```python
from build123d import *

# Parameters (mm, degrees)
F0_R     = 3.175
F1_DEPTH = 25.4


with BuildPart() as f1:
    # F0 (on Front) → F1 (new body)
    with BuildSketch(Plane.XZ):
        with BuildLine():
            Line((0.6773435479, -9.500885786), (0, -9.525))
            ThreePointArc((0, -9.525), (0.3388863295, -9.5189695375), (0.6773435479, -9.500885786))
        make_face()
        with BuildLine():
            Line((-15.7942028036, 61.9003804205), (-9.525, 0))
            ThreePointArc((-9.525, 0), (-6.7351920908, 6.7351920908), (0, 9.525))
            Line((0, 9.525), (0, 47.625))
            ThreePointArc((0, 47.625), (-10.644756084, 51.722700101), (-15.7942028036, 61.9003804205))
        make_face()
        with BuildLine():
            ThreePointArc((9.525, 0), (6.9705567315, -6.4912990883), (0.6773435479, -9.500885786))
            Line((0.6773435479, -9.500885786), (44.7324052746, -7.9324746146))
            ThreePointArc((44.7324052746, -7.9324746146), (38.9380895153, -5.7116327839), (36.5125, 0))
            Line((36.5125, 0), (9.525, 0))
        make_face()
        with BuildLine():
            Line((0, 100.0252), (0, 79.375))
            ThreePointArc((0, 79.375), (10.5003255158, 75.40625), (15.7504882737, 65.484375))
            Line((15.7504882737, 65.484375), (9.4502929642, 115.490625))
            ThreePointArc((9.4502929642, 115.490625), (9.5063048942, 114.896483242), (9.525, 114.3))
            ThreePointArc((9.525, 114.3), (6.7351920908, 107.5648079092), (0, 104.775))
            Line((0, 104.775), (0, 100.0252))
        make_face()
        with BuildLine():
            ThreePointArc((36.5125, 0), (38.9380895153, -5.7116327839), (44.7324052746, -7.9324746146))
            ThreePointArc((44.7324052746, -7.9324746146), (50.1616327839, -5.5119104847), (52.3875, 0))
            ThreePointArc((52.3875, 0), (50.1616327839, 5.5119104847), (44.7324052746, 7.9324746146))
            ThreePointArc((44.7324052746, 7.9324746146), (38.9380895153, 5.7116327839), (36.5125, 0))
        make_face()
        with BuildLine():
            ThreePointArc((47.625, 0), (44.45, -3.175), (41.275, 0))
            ThreePointArc((41.275, 0), (44.45, 3.175), (47.625, 0))
        make_face(mode=Mode.SUBTRACT)
        with BuildLine():
            ThreePointArc((9.4502929642, 115.490625), (0, 123.825), (-9.4502929642, 115.490625))
            ThreePointArc((-9.4502929642, 115.490625), (-7.14375, 107.9998046905), (0, 104.775))
            ThreePointArc((0, 104.775), (6.7351920908, 107.5648079092), (9.525, 114.3))
            ThreePointArc((9.525, 114.3), (9.5063048942, 114.896483242), (9.4502929642, 115.490625))
        make_face()
        with BuildLine():
            ThreePointArc((3.175, 114.3), (2.2450640303, 112.0549359697), (0, 111.125))
            ThreePointArc((0, 111.125), (-2.2450640303, 116.5450640303), (3.175, 114.3))
        make_face(mode=Mode.SUBTRACT)
        with BuildLine():
            Line((0, 60.325), (0, 47.625))
            ThreePointArc((0, 47.625), (10.6492737428, 51.7267849017), (15.7954255641, 61.9125))
            ThreePointArc((15.7954255641, 61.9125), (15.8550939106, 62.7052534459), (15.875, 63.5))
            ThreePointArc((15.875, 63.5), (15.8438414904, 64.4941387366), (15.7504882737, 65.484375))
            ThreePointArc((15.7504882737, 65.484375), (10.5003255158, 75.40625), (0, 79.375))
            Line((0, 79.375), (0, 66.675))
            ThreePointArc((0, 66.675), (2.2450640303, 65.7450640303), (3.175, 63.5))
            ThreePointArc((3.175, 63.5), (2.2450640303, 61.2549359697), (0, 60.325))
        make_face()
        with BuildLine():
            ThreePointArc((-15.7504882737, 65.484375), (-15.8738192656, 63.6936154008), (-15.7942028036, 61.9003804205))
            ThreePointArc((-15.7942028036, 61.9003804205), (-10.644756084, 51.722700101), (0, 47.625))
            Line((0, 47.625), (0, 60.325))
            ThreePointArc((0, 60.325), (-3.175, 63.5), (0, 66.675))
            Line((0, 66.675), (0, 79.375))
            ThreePointArc((0, 79.375), (-10.5003255158, 75.40625), (-15.7504882737, 65.484375))
        make_face()
        with BuildLine():
            Line((0, 47.625), (0, 9.525))
            ThreePointArc((0, 9.525), (6.7351920908, 6.7351920908), (9.525, 0))
            Line((9.525, 0), (36.5125, 0))
            ThreePointArc((36.5125, 0), (38.9380895153, 5.7116327839), (44.7324052746, 7.9324746146))
            Line((44.7324052746, 7.9324746146), (18.968327868, 8.8497055806))
            ThreePointArc((18.968327868, 8.8497055806), (13.2612039825, 11.5674628959), (11.3408358685, 17.5898921545))
            Line((11.3408358685, 17.5898921545), (15.7954255641, 61.9125))
            ThreePointArc((15.7954255641, 61.9125), (10.6492737428, 51.7267849017), (0, 47.625))
        make_face()
        with BuildLine():
            ThreePointArc((0, 9.525), (-6.7351920908, 6.7351920908), (-9.525, 0))
            ThreePointArc((-9.525, 0), (-6.7351920908, -6.7351920908), (0, -9.525))
            Line((0, -9.525), (0.6773435479, -9.500885786))
            ThreePointArc((0.6773435479, -9.500885786), (6.9705567315, -6.4912990883), (9.525, 0))
            Line((9.525, 0), (3.175, 0))
            ThreePointArc((3.175, 0), (-2.2450640303, -2.2450640303), (0, 3.175))
            Line((0, 3.175), (0, 9.525))
        make_face()
        with BuildLine():
            ThreePointArc((9.525, 0), (6.7351920908, 6.7351920908), (0, 9.525))
            Line((0, 9.525), (0, 3.175))
            ThreePointArc((0, 3.175), (2.2450640303, 2.2450640303), (3.175, 0))
            Line((3.175, 0), (9.525, 0))
        make_face()
        with BuildLine():
            Line((-9.4502929642, 115.490625), (-15.7504882737, 65.484375))
            ThreePointArc((-15.7504882737, 65.484375), (-10.5003255158, 75.40625), (0, 79.375))
            Line((0, 79.375), (0, 100.0252))
            Line((0, 100.0252), (0, 104.775))
            ThreePointArc((0, 104.775), (-7.14375, 107.9998046905), (-9.4502929642, 115.490625))
        make_face()
        with Locations((-3.175, 100.0252)):
            Circle(F0_R, mode=Mode.SUBTRACT)
    extrude(amount=F1_DEPTH)


solid = f1.part
```
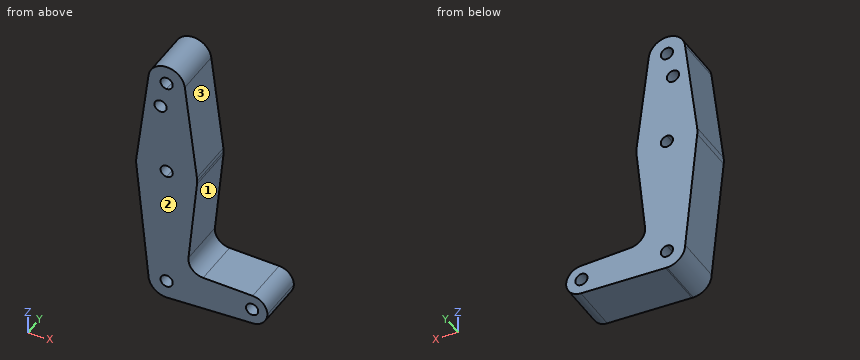
Check sheet for the modelled part. Datum: model origin and axes. Units: mm. Face numbers are marked on the shaded views. Round coordinates to 2 decimals unless told otherwise and drop trailing zeros. Order: outer loops, then holes, each group sorted by start corner. A loop starts at its lowest first (then second) coordinate and runs counter-clockwise, first axis right, second up.
1) Section check C-C (x = 36). Record the boundary of the cut face in (y, z), and give its area (3 significant figures).
2) Go/stop test with flat-tipped pins: pin 1 Ø6 at (x, y) = (4.5, -3.5) entering from -Z; pin 2 Ø5.5 at (x, z) = (44.45, 0) entering from +Y; pin 3 Ø1 at (x, y) = (4, -20.5) entering from -Z; pin 4 Ø4 at (x, y) = (21, -16.5) entering from +Z. Record where each tip stops, or that it passes through.
3) Scan lines: line 1 (Z direction, x = 44.45, y = -6.5) (3 decimals); line 2 (Z direction, x = 2, y = -10.5); line 3 (X direction, y = -15.75, z = -1.5). Record each from-to range of solid material in increasing order.
4) Section check B-B (z = 6). Record the boundary of the cut face in (x, y).
5) Mould release check, pull along Z, two halves, no side actions. Record for the marked faces 1, 2 and 3: +Z half, -Z half, draft (parallel to the pull), parting line (faces both ways), or undercut.
6) Section check A-A (y = -11.25). Give the number of separate pieces and of enclosed holes in the cut face, and give its area (3 significant figures).
Result:
1. outline: (-25.4, -8.24) - (0, -8.24) - (0, 8.24) - (-25.4, 8.24) - close
1. area: 419 mm2
2. pin 1: stops at z = -9.47
2. pin 2: passes through
2. pin 3: stops at z = -9.4
2. pin 4: stops at z = 8.85
3. line 1: z = -7.943 to -3.175, 3.175 to 7.943
3. line 2: z = -9.45 to -2.47, 2.47 to 61.03, 65.97 to 111.83, 116.77 to 123.61
3. line 3: x = -9.41 to -2.8, 2.8 to 41.65, 47.25 to 52.24
4. outline: (-10.13, -25.4) - (49.65, -25.4) - (49.65, 0) - (-10.13, 0) - close
5. face 1: undercut
5. face 2: draft
5. face 3: +Z half
6. separate pieces: 1
6. enclosed holes: 5
6. area: 3,770 mm2
